from build123d import *

# Parameters (mm, degrees)
SKETCH1_W               = 225.425
SKETCH1_H               = 100.69322
BOSS_EXTRUDE1_DEPTH     = 24.35352
SKETCH2_W               = 6.35
SKETCH2_H               = 24.385376466
BOSS_EXTRUDE2_DEPTH     = 100.69322
SKETCH3_W               = 6.35
SKETCH3_H               = 24.35352
BOSS_EXTRUDE3_DEPTH     = 100.69322
SKETCH4_R               = 12.64539
SKETCH4_R_2             = 10.58672
CUT_EXTRUDE1_DEPTH      = 254.873726713
CUT_EXTRUDE2_DEPTH      = 254.876784611
CUT_EXTRUDE2_DEPTH_BACK = 254.876784611
SKETCH16_R              = 31.75
SKETCH16_R_2            = 24.765
CUT_EXTRUDE6_DEPTH      = 12.17676
SKETCH17_R              = 24.765
CUT_EXTRUDE7_DEPTH      = 254.873726713


with BuildPart() as part:
    # Sketch1 → Boss-Extrude1 (new body)
    with BuildSketch(Plane(origin=(0, 0, 0), x_dir=(1, 0, 0), z_dir=(0, 1, 0))):
        with Locations((112.7125, 50.34661)):
            Rectangle(SKETCH1_W, SKETCH1_H)
    extrude(amount=BOSS_EXTRUDE1_DEPTH)

    # Sketch2 → Boss-Extrude2 (add)
    with BuildSketch(Plane.XY.offset(-100.69322)):
        with Locations((-3.175, 12.192688233)):
            Rectangle(SKETCH2_W, SKETCH2_H)
    extrude(amount=BOSS_EXTRUDE2_DEPTH)

    # Sketch3 → Boss-Extrude3 (add)
    with BuildSketch(Plane(origin=(225.425, 0, -100.69322), x_dir=(-1, 0, 0), z_dir=(0, 0, -1))):
        with Locations((-3.175, 12.17676)):
            Rectangle(SKETCH3_W, SKETCH3_H)
    extrude(amount=-BOSS_EXTRUDE3_DEPTH)

    # Sketch4 → Cut-Extrude1 (cut, through all)
    with BuildSketch(Plane(origin=(0, 24.35352, 0), x_dir=(1, 0, 0), z_dir=(0, 1, 0))):
        with Locations(Location((17.2085, 76.49718, 0), (0, 0, 270))):
            Circle(SKETCH4_R)
        with Locations(Location((145.99666, 84.074, 0), (0, 0, 270))):
            Circle(SKETCH4_R_2)
    extrude(amount=-CUT_EXTRUDE1_DEPTH, mode=Mode.SUBTRACT)

    # Sketch5 → Cut-Extrude2 (cut, two sides: drawn at the far end of the back side and taken through both)
    with BuildSketch(Plane(origin=(0, 24.385376466, 0), x_dir=(1, 0, 0), z_dir=(0, 1, 0)).offset(-CUT_EXTRUDE2_DEPTH_BACK)):
        Polygon((-509.055541284, -36.086678247), (-6.35, 88.139743453), (44.45, 100.69322), (547.155541284, 224.9196417), (298.702697883, 1230.330724268), (-757.508384685, 969.324404321), align=None)
    extrude(amount=CUT_EXTRUDE2_DEPTH + CUT_EXTRUDE2_DEPTH_BACK, mode=Mode.SUBTRACT)

    # Sketch16 → Cut-Extrude6 (cut)
    with BuildSketch(Plane(origin=(0, 24.35352, 0), x_dir=(1, 0, 0), z_dir=(0, 1, 0))):
        with Locations(Location((104.78262, 51.0794, 0), (0, 0, 270))):
            Circle(SKETCH16_R)
        with Locations(Location((104.78262, 51.0794, 0), (0, 0, 270))):
            Circle(SKETCH16_R_2, mode=Mode.SUBTRACT)
    extrude(amount=-CUT_EXTRUDE6_DEPTH, mode=Mode.SUBTRACT)

    # Sketch17 → Cut-Extrude7 (cut, through all)
    with BuildSketch(Plane(origin=(0, 24.35352, 0), x_dir=(1, 0, 0), z_dir=(0, 1, 0))):
        with Locations(Location((104.78262, 51.0794, 0), (0, 0, 270))):
            Circle(SKETCH17_R)
    extrude(amount=-CUT_EXTRUDE7_DEPTH, mode=Mode.SUBTRACT)


solid = part.part
Read the model definition and answer for the solid it produces. Units are mm, in the model's axes. A direction names the side the tool comes from. Give positions to 0.01 mm unless a question says otherwise; leave off trailing zeros. Write each loop counter-clockwise with the first axis right and the second up, starting at its lowest first coordinate (ties: lowest second). Pieces come first, ordered by that corner, then holes. Notation, with made-up numbers: (33, 25) - (90, 25) arc R26 ccw to (90, 42) - close; hole circle Ø8 at (42.25, -24.5). An arc over 180 degrees is marked (long way). Answer in a Markdown table with one row per item. Add a question column.
Item 1: Section A-A, the plane x = 120 is taken. Write down the section's boundary in (y, z), and give its area (3 significant figures).
Item 2: A tool of negligible diameter and unlimited length cuts with its end or side. For faces 1 (the face through (105.87, 6.17, -75.82)), 2 (the face through (88, 12.177, -32)), from which of +Z, -Z, +X, -X, +Y, -Y can it reach the whole face along a straight path? Write none if from no direction.
Item 3: Section D-D, the plane z = -68 is taken. Write down the section's boundary in (x, y) (3 decimals).
Item 4: Section B-B, the plane z = -30 is taken. Write down the section's boundary in (x, y) (3 decimals), and give its area (3 significant figures).
Item 5: Section C-C, the plane y = 6.5 is taken. Count the separate pieces of the cut face and the enclosed holes in it, and give its area (3 significant figures).
Item 6: Find the intervals of material crossed by L1, parallel to X at y = 17, z = -67.5 (3 decimals); L2, parallel to X at y = 14, z = -67 (3 decimals); L3, parallel to Z at x = 146, y = 16, in increasing order.
Item 7: Determine the mould class of faces 3 (the face through (-6.35, 12, -45)), 4 (the face through (231.775, 12, -51)), 5 (the face through (21.007, 12.347, -64.436)), 6 (the face through (-3, 24.385, -45)) for opening direction X: pulls with the +X half, pulls with the -X half, needs draft (parallel to the pull), parting line crosses it, or undercut.
Item 8: A flat-ended cylindrical pin translates along its axis: P1, Ø8, axis at x = 156, y = 19.5, coming from the +Z side. Find the tip coordinate at first contact, or state that the pin passes through.
Recorded:
| question | item | result |
|---|---|---|
| 1 | outline | (0, -100.69) - (24.35, -100.69) - (24.35, -78.95) - (12.18, -78.95) - (12.18, -70.62) - (0, -70.62) - close; (0, -31.54) - (12.18, -31.54) - (12.18, -23.21) - (24.35, -23.21) - (24.35, 0) - (0, 0) - close |
| 1 | area | 1,300 mm2 |
| 2 | face 1 | +Y, -Y |
| 2 | face 2 | +Y |
| 3 | outline | (-6.35, 0) - (7.843, 0) - (7.843, 24.354) - (0, 24.354) - (0, 24.385) - (-6.35, 24.385) - close; (26.574, 0) - (86.7, 0) - (86.7, 12.177) - (77.917, 12.177) - (77.917, 24.354) - (26.574, 24.354) - close; (122.866, 0) - (231.775, 0) - (231.775, 24.354) - (131.648, 24.354) - (131.648, 12.177) - (122.866, 12.177) - close |
| 4 | outline | (-6.35, 0) - (91.784, 0) - (91.784, 12.177) - (81.04, 12.177) - (81.04, 24.354) - (0, 24.354) - (0, 24.385) - (-6.35, 24.385) - close; (117.781, 0) - (231.775, 0) - (231.775, 24.354) - (128.525, 24.354) - (128.525, 12.177) - (117.781, 12.177) - close |
| 4 | area | 4,900 mm2 |
| 5 | separate pieces | 1 |
| 5 | enclosed holes | 3 |
| 5 | area | 20,900 mm2 |
| 6 | L1 | x = -6.35 to 8.323, 26.094 to 77.609, 131.957 to 231.775 |
| 6 | L2 | x = -6.35 to 8.859, 25.558 to 77.313, 132.253 to 231.775 |
| 6 | L3 | z = -100.69 to -94.66, -73.49 to 0 |
| 7 | face 3 | pulls with the -X half |
| 7 | face 4 | pulls with the +X half |
| 7 | face 5 | undercut |
| 7 | face 6 | needs draft |
| 8 | P1 | stops at z = 0 |
